Geometry check sheet. Reference: the model listing, model coordinates, mm. A direction names the side the tool comes from. Give positions to 0.01 mm unless a question says otherwise; leave off trailing zeros. Loops run counter-clockwise (first coordinate to the right, second up) from the corner with the lowest first, then second, coordinate; pieces in that order, holes last. Notation, with made-up numbers: (62.5, 47) -> (68.5, 47) arc R14 ccw to (68.5, 71) -> close; hole circle Ø10 at (3, -9). An arc over 180 degrees is marked (long way). Answer in a Markdown table with one row per item. Add a question column.
```python
from build123d import *

# Parameters (mm, degrees)
SKETCH1_W             = 180
SKETCH1_H             = 35
BOSS_EXTRUDE1_DEPTH   = 5
F_6_0MM_DOWEL_HOLE1_D = 6
SKETCH4_W             = 160
SKETCH4_H             = 35
CUT_EXTRUDE1_DEPTH    = 2
CHAMFER1_SIZE         = 10


with BuildPart() as part:
    # Sketch1 → Boss-Extrude1 (new body)
    with BuildSketch(Plane(origin=(0, 0, 0), x_dir=(1, 0, 0), z_dir=(0, 1, 0))):
        Rectangle(SKETCH1_W, SKETCH1_H)
    extrude(amount=BOSS_EXTRUDE1_DEPTH)

    # Ø6.0mm Dowel Hole1 (through all)
    with Locations(Plane(origin=(-60, 5, -6.25), x_dir=(0, 0, 1), z_dir=(0, 1, 0))):
        with Locations((0, 0), (17.5, 0), (0, 120), (17.5, 120)):
            Hole(F_6_0MM_DOWEL_HOLE1_D / 2)

    # Sketch4 → Cut-Extrude1 (cut)
    with BuildSketch(Plane(origin=(0, 5, 0), x_dir=(1, 0, 0), z_dir=(0, 1, 0))):
        Rectangle(SKETCH4_W, SKETCH4_H)
    extrude(amount=-CUT_EXTRUDE1_DEPTH, mode=Mode.SUBTRACT)

    # Chamfer1
    chamfer1_edges = [part.edges().sort_by_distance(p)[0] for p in [
        (90, 2.5, -17.5),
        (-90, 2.5, -17.5),
    ]]
    chamfer(chamfer1_edges, length=CHAMFER1_SIZE)


solid = part.part
```
1. Release check for a two-part mould opening along X. For faces 1 (the face through (85.1, 2.5, -12.4)), 2 (the face through (-90, 2, 5)), 3 (the face through (62.974, 1.479, -5.859)), 4 (the face through (-85, 5, 4)) record: released by +X, released by -X, zero draft, split by the parting line, or undercut.
2. Gauge pin test, flat end, axial feed: pin 1 Ø3.5 at (x, z) = (-60, 11.25) entering from +Y. Record the tip position at first contact, or that the pin passes through.
3. Sectioned sample at D-D (z = -0.5). Enter the section's corners in (x, y), plus the area to 3 significant figures.
4. Access from +Z, -Z, +X, -X, +Y, -Y to the whole of each face (thin tool, end or side, straight path). Record for faces 5 (the face through (-1, 0, 0)), 6 (the face through (-1, 3, 0)).
5. Sectioned sample at B-B (x = 60). Enter the section's corners in (y, z), plus the area to 3 significant figures.
6. Sectioned sample at A-A (z = 11.25). Enter the section's corners in (x, y).
7. Material ranges on L1, parallel to X at y = 1.55, z = -6.25; L2, parallel to X at y = 3.4, z = 9; L3, parallel to X at y = 0.95, z = -8, recorded low to high. Write a range as from..to.
8. Sectioned sample at C-C (y = 4.1). Enter the section's corners in (x, z).
Response:
| question | item | result |
|---|---|---|
| 1 | face 1 | released by +X |
| 1 | face 2 | released by -X |
| 1 | face 3 | undercut |
| 1 | face 4 | zero draft |
| 2 | pin 1 | passes through |
| 3 | outline | (-90, 0) -> (90, 0) -> (90, 5) -> (80, 5) -> (80, 3) -> (-80, 3) -> (-80, 5) -> (-90, 5) -> close |
| 3 | area | 580 mm2 |
| 4 | face 5 | +Z, -Z, +X, -X, -Y |
| 4 | face 6 | +Z, -Z, +Y |
| 5 | outline | (0, -17.5) -> (3, -17.5) -> (3, -9.25) -> (0, -9.25) -> close; (0, -3.25) -> (3, -3.25) -> (3, 8.25) -> (0, 8.25) -> close; (0, 14.25) -> (3, 14.25) -> (3, 17.5) -> (0, 17.5) -> close |
| 5 | area | 69.0 mm2 |
| 6 | outline | (-90, 0) -> (-63, 0) -> (-63, 3) -> (-80, 3) -> (-80, 5) -> (-90, 5) -> close; (-57, 0) -> (57, 0) -> (57, 3) -> (-57, 3) -> close; (63, 0) -> (90, 0) -> (90, 5) -> (80, 5) -> (80, 3) -> (63, 3) -> close |
| 7 | L1 | x = -90..-63, -57..57, 63..90 |
| 7 | L2 | x = -90..-80, 80..90 |
| 7 | L3 | x = -89.5..-62.44, -57.56..57.56, 62.44..89.5 |
| 8 | outline | (-90, -7.5) -> (-80, -17.5) -> (-80, 17.5) -> (-90, 17.5) -> close; (80, -17.5) -> (90, -7.5) -> (90, 17.5) -> (80, 17.5) -> close |
